from build123d import *

# Parameters (mm, degrees)
BOSS_EXTRUDE1_DEPTH = 375


with BuildPart() as part:
    # Master sketch-Wing Geometry Master Sketc → Boss-Extrude1 (new body)
    with BuildSketch(Plane.XY):
        with BuildLine():
            Line((299.93, -0.56), (300.07, 0.56))
            add(Edge.make_bspline(
                [(300.07, 0.56), (300.046727211, 0.570149465), (299.951918411, 0.611496405), (299.73145109, 0.687910176), (299.360701306, 0.80207776), (298.851143071, 0.99004976), (298.192762058, 1.214989557), (297.390581316, 1.498347711), (296.440162644, 1.827131445), (295.347552696, 2.205915898), (294.109915848, 2.626416664), (292.734867315, 3.097875543), (291.212205014, 3.603301609), (289.556778296, 4.170360104), (287.754541524, 4.750229424), (285.826587723, 5.399922294), (283.756363975, 6.062421055), (281.558560221, 6.775887077), (279.22562543, 7.517307408), (276.759052146, 8.280298176), (274.172767845, 9.09557711), (271.459553567, 9.926240206), (268.620233525, 10.77076618), (265.667031068, 11.655929728), (262.589976024, 12.539934752), (259.406507793, 13.464429613), (256.106091201, 14.393267862), (252.694259979, 15.330032696), (249.183398904, 16.29260897), (245.565461503, 17.251434656), (241.852861879, 18.22108263), (238.042855476, 19.19138103), (234.140998952, 20.15735732), (230.154027103, 21.143304457), (227.071354515, 21.873459433), (225.320067796, 22.282419133), (224.93, 22.373189537)],
                knots=[0, 0, 0, 0, 0.000121802, 0.000496198, 0.001118298, 0.001983272, 0.003101095, 0.004456671, 0.0060651, 0.00792639, 0.010005101, 0.012336683, 0.014900868, 0.017702772, 0.020732285, 0.023984296, 0.027464026, 0.031161268, 0.035071154, 0.039209025, 0.043549161, 0.048082096, 0.052823294, 0.05776212, 0.062874254, 0.068184085, 0.073667486, 0.07932465, 0.085159937, 0.091134213, 0.09728269, 0.103570554, 0.109998008, 0.116569035, 0.123276218, 0.125197771, 0.125197771, 0.125197771, 0.125197771], degree=3))
            Line((224.93, 22.373189537), (240.711180377, -4.960616679))
            add(Edge.make_bspline(
                [(240.711180377, -4.960616679), (241.664163028, -4.887637656), (243.840258172, -4.718440324), (247.20981219, -4.46085993), (250.787106765, -4.195760616), (254.266072169, -3.918835614), (257.64325016, -3.672183933), (260.913793207, -3.436175985), (264.072684975, -3.187909636), (267.117194027, -2.977146375), (270.04316125, -2.751013416), (272.846765874, -2.544700113), (275.529429199, -2.33878816), (278.087148077, -2.166666674), (280.513268395, -1.982425314), (282.806745266, -1.814435769), (284.962823137, -1.649552143), (286.983837234, -1.517010694), (288.863257365, -1.37227381), (290.600165156, -1.245587565), (292.192790163, -1.119159502), (293.640594786, -1.028164187), (294.939565333, -0.920704317), (296.089960301, -0.842870725), (297.090587221, -0.777681987), (297.939585238, -0.701301857), (298.63665195, -0.653077401), (299.177018782, -0.618208827), (299.562595702, -0.575799674), (299.797349193, -0.578243239), (299.903360171, -0.56366373), (299.93, -0.56)],
                knots=[0.905027219, 0.905027219, 0.905027219, 0.905027219, 0.909613035, 0.915499668, 0.921241563, 0.92682399, 0.932244523, 0.93748843, 0.942556897, 0.947447555, 0.952130861, 0.956637537, 0.960935685, 0.965040102, 0.968937144, 0.972609709, 0.976073746, 0.979312161, 0.982327244, 0.985117851, 0.987668032, 0.989992582, 0.992077865, 0.99392155, 0.995524803, 0.996888844, 0.998011233, 0.998877243, 0.999486883, 0.999871057, 1, 1, 1, 1], degree=3))
        make_face()
        Polygon((277.5184867, 2.809088635), (243.466590848, 0.266872389), (235.093272506, 14.769885184), align=None, mode=Mode.SUBTRACT)
    extrude(amount=BOSS_EXTRUDE1_DEPTH)


solid = part.part
Geometry check sheet. Reference: the model listing, model coordinates, mm. Give positions to 0.01 mm unless a question says otherwise; leave off trailing zeros. Use a Markdown table: item, result.
Item 1: Material ranges on line 1 along Y through (x, z) = (250, 205); line 2 along Y through (x, z) = (274, 116); line 3 along Y through (x, z) = (289.5, 186.5), recorded low to high.
Answers follow:
| item | result |
|---|---|
| line 1 | y = -4.25 to 0.75, 10.57 to 16.07 |
| line 2 | y = -2.46 to 2.55, 3.8 to 9.15 |
| line 3 | y = -1.33 to 4.18 |
Item 2: Draft check along Y on faces 1 (the flat face through (232.71, 8.9, 184.88)), 2 (the flat face through (256.009, 8.873, 184.875)), 3 (the flat face through (257, 11, 375)). Enter one of: +Y half, -Y half, draft (parallel to the pull), parting line (faces both ways), or undercut.
Answers follow:
| item | result |
|---|---|
| face 1 | -Y half |
| face 2 | undercut |
| face 3 | draft |
Item 3: Depth check by flat-ended pin: P1, Ø1, axis at x = 234, z = 259, coming from the -Y side; P2, Ø12, axis at y = 3, z = 75.5, coming from the -X side; P3, Ø6, axis at x = 263.5, z = 218.5, coming from the -Y side. Enter the tip coordinate at first touch or a pass-through.
Answers follow:
| item | result |
|---|---|
| P1 | stops at y = 5.8 |
| P2 | stops at x = 232.65 |
| P3 | stops at y = -3.46 |
